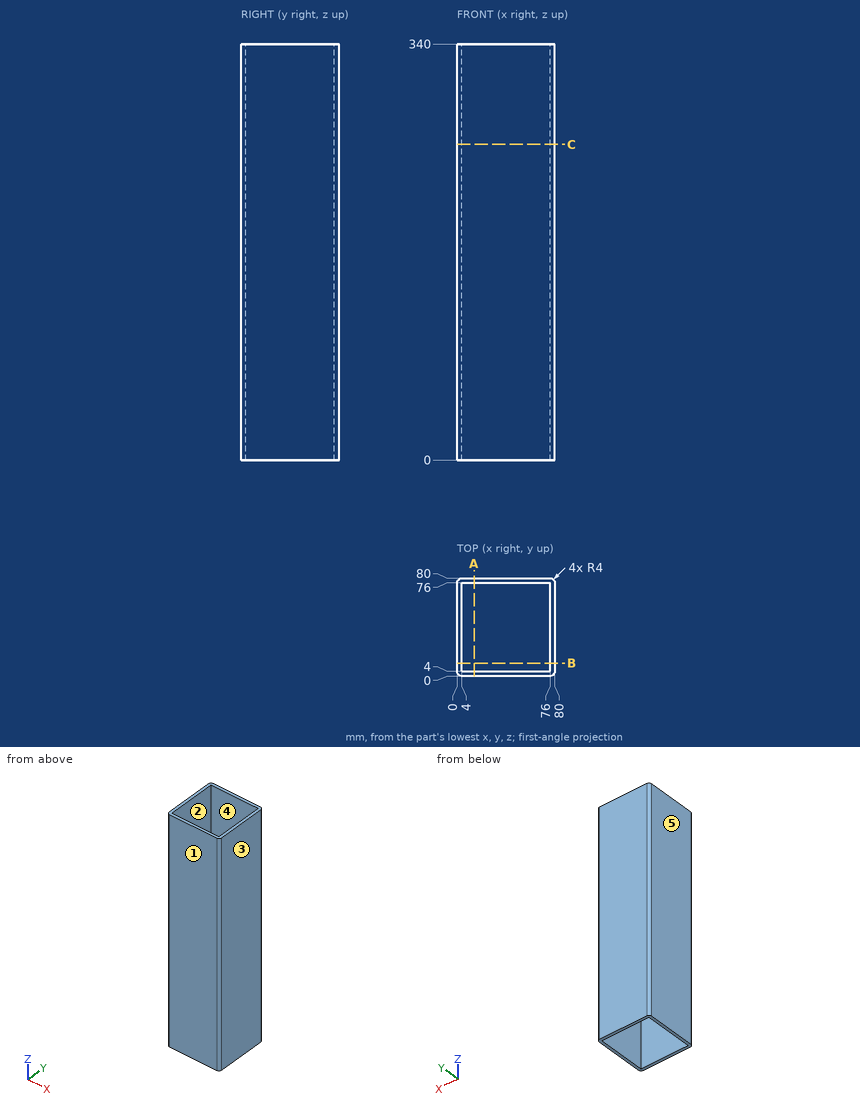
Drawing for the job (mm, zero at the part's lowest x, y, z). A direction names the side the tool comes from. Give positions to 0.01 mm unless a question says otherwise; leave off trailing zeros. Loops run counter-clockwise (first coordinate to the right, second up) from the corner with the lowest first, then second, coordinate; pieces in that order, holes last. Notation, with made-up numbers: M 85.5,79 L 103.5,79 A23 ccw 103.5,90 Z; hole C 51.5,-29.75 d11. An arc over 180 degrees is marked long. One line per question, with ' | ' between items. Start each with the question number.
1. Probe L1, parallel to X at y = 11, z = 49.5. List the from-to ranges inside material, lowest first. Write a range as from..to.
2. Two-plate mould, pull along X, no slides. Class the marked faces 1, 2 and 3: pulls with the +X half, pulls with the -X half, needs draft (parallel to the pull), parting line crosses it, or undercut.
3. Saw through at A-A on x = 14. Give the cut face in (y, z), plus the area to 3 significant figures.
4. Saw through at C-C on z = 258. Give the cut face in (x, y).
5. 3-axis set-ups, long thin cutter, end or side, ignore diameter. For the marked faces 4 and 5: which of +Z, -Z, +X, -X, +Y, -Y reach the whole face in a straight line?
Result sheet:
1) L1: x = 0..4, 76..80
2) face 1: needs draft | face 2: undercut | face 3: pulls with the +X half
3) outline: M 0,0 L 4,0 L 4,340 L 0,340 Z; M 76,0 L 80,0 L 80,340 L 76,340 Z | area: 2,720 mm^2
4) outline: M 0,4 A4 ccw 4,0 L 76,0 A4 ccw 80,4 L 80,76 A4 ccw 76,80 L 4,80 A4 ccw 0,76 Z; hole M 4,4 L 76,4 L 76,76 L 4,76 Z
5) face 4: +Z, -Z | face 5: +Z, -Z, -X, +Y, -Y
